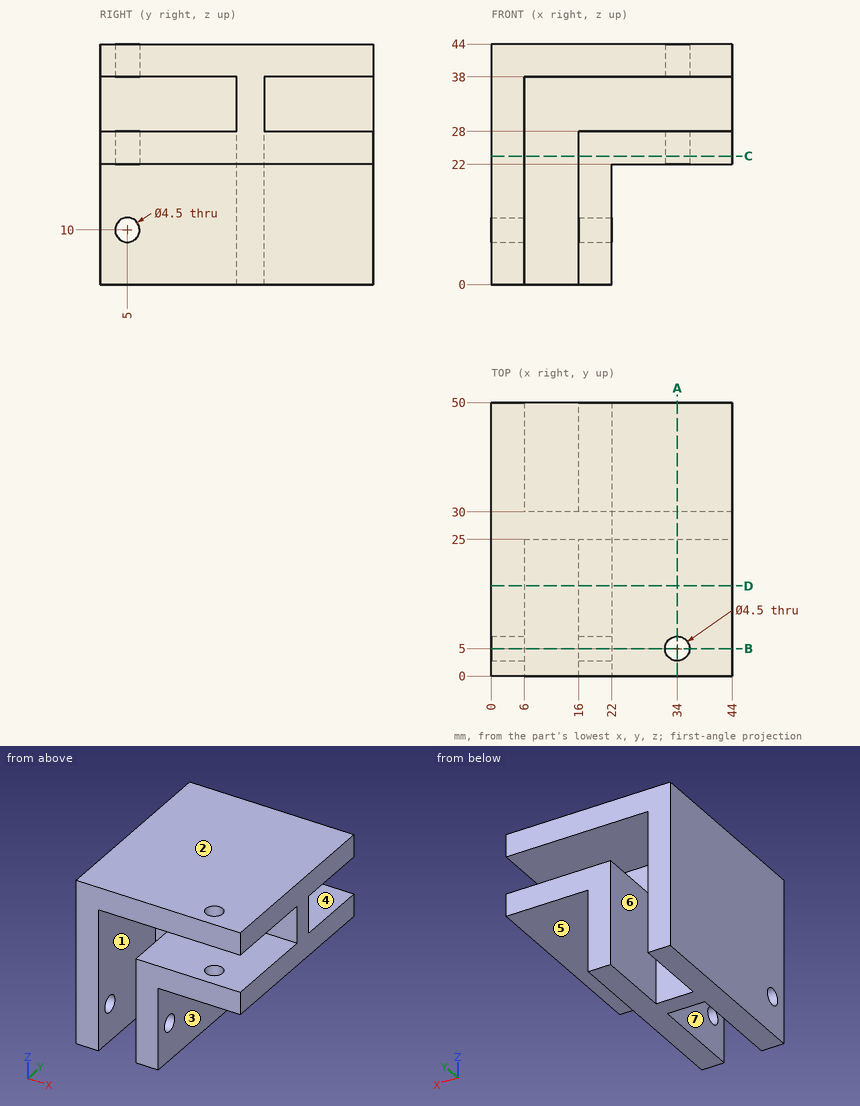
Design review of the part shown in the three views and the two pictorial views. Dimensions are in mm from the part's minimum x, y and z. A direction names the side the tool comes from. Give positions to 0.01 mm unless a question says otherwise; leave off trailing zeros. Write each loop counter-clockwise with the first axis right and the second up, starting at its lowest first coordinate (ties: lowest second). Pieces come first, ordered by that corner, then holes.
Item 1: Machinability: for the marked faces 4, 5, 6 and 7, which of the approach directions +Z, -Z, +X, -X, +Y, -Y give a long, thin tool a straight path to every point of the face, cutting with its end or side? Answer none if there is none.
Item 2: Take a section at D-D (y = 16.5). Give the boundary of the cut face in (x, z), and give its area (3 significant figures).
Item 3: Take a section at A-A (x = 34). Give the boundary of the cut face in (y, z).
Item 4: Take a section at B-B (y = 5). Give the boundary of the cut face in (x, z).
Item 5: The part is to be moulded in two halves that separate along X. For the marked faces 1, 2 and 3, say which applies: +X half, -X half, draft (parallel to the pull), parting line (faces both ways), or undercut.
Item 6: Wall thickness on probe 1 along Y at (x, z) = (2.3, 10); probe 2 along X at (y, z) = (34.5, 13); probe 3 along Z at (x, y) = (21.5, 7.5): over which ranges is each line inside the solid? List them lowest first.
Item 7: Take a section at C-C (z = 23.5). Give the boundary of the cut face in (x, y).
Item 8: Insertion check: P1, Ø8, axis at x = 12.5, z = 30.5, coming from the -Y side; P2, Ø20, axis at y = 12, z = 16.5, coming from the -X side; P3, Ø11, axis at x = 38, y = 17.5, coming from the -Z side; P4, Ø6.5, axis at y = 27.5, z = 12, coming from the +X side. Each pin has a flat end and moves straight along its axis. Give the tip position at first contact, or say it passes through.
Established:
1. face 4: +X, +Y
1. face 5: -Z, +X, +Y, -Y
1. face 6: -Z, +Y
1. face 7: -Z, -Y
2. outline: (0, 0) - (6, 0) - (6, 38) - (44, 38) - (44, 44) - (0, 44) - close; (16, 0) - (22, 0) - (22, 22) - (44, 22) - (44, 28) - (16, 28) - close
2. area: 792 mm2
3. outline: (0, 22) - (2.75, 22) - (2.75, 28) - (0, 28) - close; (0, 38) - (2.75, 38) - (2.75, 44) - (0, 44) - close; (7.25, 22) - (50, 22) - (50, 28) - (30, 28) - (30, 38) - (50, 38) - (50, 44) - (7.25, 44) - (7.25, 38) - (25, 38) - (25, 28) - (7.25, 28) - close
4. outline: (0, 0) - (6, 0) - (6, 7.75) - (0, 7.75) - close; (0, 12.25) - (6, 12.25) - (6, 38) - (31.75, 38) - (31.75, 44) - (0, 44) - close; (16, 0) - (22, 0) - (22, 7.75) - (16, 7.75) - close; (16, 12.25) - (22, 12.25) - (22, 22) - (31.75, 22) - (31.75, 28) - (16, 28) - close; (36.25, 22) - (44, 22) - (44, 28) - (36.25, 28) - close; (36.25, 38) - (44, 38) - (44, 44) - (36.25, 44) - close
5. face 1: undercut
5. face 2: draft
5. face 3: +X half
6. probe 1: y = 0 to 2.75, 7.25 to 50
6. probe 2: x = 0 to 6, 16 to 22
6. probe 3: z = 0 to 28, 38 to 44
7. outline: (0, 0) - (6, 0) - (6, 25) - (16, 25) - (16, 0) - (44, 0) - (44, 50) - (16, 50) - (16, 30) - (6, 30) - (6, 50) - (0, 50) - close; hole circle Ø4.5 at (34, 5)
8. P1: stops at y = 25
8. P2: stops at x = 0
8. P3: stops at z = 22
8. P4: stops at x = 22
